Read the model definition and answer for the solid it produces. Units are mm, in the model's axes. Coordinates: 2 decimals unless noted, no trailing zeros. Write each loop counter-clockwise with the first axis right and the second up, starting at its lowest first coordinate (ties: lowest second). Pieces come first, ordered by that corner, then holes. Notation, with made-up numbers: (80, 44.25) -> (118, 44.25) arc R19 ccw to (118, 80.25) -> close; hole circle Ø1 at (12.25, -13). An arc over 180 degrees is marked (long way). One line per item, written item: value. Start each with the question number.
1. Find section B-B, the plane x = -12.7. Write down the section's boundary in (y, z).
2. Find section A-A, the plane y = 0. Write down the section's boundary in (x, z).
3. For a pull along Y with two mould halves and no side action, classify faces 1 (the flat face through (0, -25.4, -3)), 2 (the flat face through (0, 25.4, -3)), 3 (the cylindrical face through (-9.59, 2.85, -5.4)), 4 (the flat face through (0, 0, 0)) as pulls with the +Y half, pulls with the -Y half, needs draft (parallel to the pull), parting line crosses it, or undercut.
4. Consider line 1 along X through (y, z) = (0, -4.75); line 2 along Y through (x, z) = (-12.7, -5.7); line 3 along X through (y, z) = (4, -2). Determine where each line is inside the solid, lowest interval first.
5. Find section C-C, the plane z = -1.25. Write down the section's boundary in (x, y), and give its area (3 significant figures).
6. Given P1, Ø13.5, axis at x = -12.7, y = 0, coming from the -Z side; P2, Ø5, axis at x = 12.7, y = 0, coming from the +Z side, each flat-ended and moving along its own axis, determine where each tip first touches the part or whether it passes through.
```python
from build123d import *

# Parameters (mm, degrees)
SKETCH1_W                                         = 50.8
SKETCH1_H                                         = 50.8
SKETCH1_R                                         = 3.2639
BOSS_EXTRUDE1_DEPTH                               = 6.35
CSK_FOR_5_16_FLAT_HEAD_MACHINE_SCREW1_D           = 8.4328
CSK_FOR_5_16_FLAT_HEAD_MACHINE_SCREW1_DEPTH       = 32.766
CSK_FOR_5_16_FLAT_HEAD_MACHINE_SCREW1_CSINK_D     = 16.129
CSK_FOR_5_16_FLAT_HEAD_MACHINE_SCREW1_CSINK_ANGLE = 82
CSK_FOR_5_16_FLAT_HEAD_MACHINE_SCREW1_TIP         = 2.533468714


with BuildPart() as part:
    # Sketch1 → Boss-Extrude1 (new body)
    with BuildSketch(Plane.XY):
        Rectangle(SKETCH1_W, SKETCH1_H)
        with Locations((-12.7, 0)):
            Circle(SKETCH1_R, mode=Mode.SUBTRACT)
        with Locations((12.7, 0)):
            Circle(SKETCH1_R, mode=Mode.SUBTRACT)
    extrude(amount=-BOSS_EXTRUDE1_DEPTH)

    # CSK for 5/16 Flat Head Machine Screw1
    with Locations(Plane(origin=(-12.7, 0, 0), x_dir=(1, 0, 0), z_dir=(0, 0, 1))):
        with Locations((0, 0), (25.4, 0)):
            CounterSinkHole(CSK_FOR_5_16_FLAT_HEAD_MACHINE_SCREW1_D / 2, CSK_FOR_5_16_FLAT_HEAD_MACHINE_SCREW1_CSINK_D / 2, depth=CSK_FOR_5_16_FLAT_HEAD_MACHINE_SCREW1_DEPTH, counter_sink_angle=CSK_FOR_5_16_FLAT_HEAD_MACHINE_SCREW1_CSINK_ANGLE)
            with Locations((0, 0, -(CSK_FOR_5_16_FLAT_HEAD_MACHINE_SCREW1_DEPTH + CSK_FOR_5_16_FLAT_HEAD_MACHINE_SCREW1_TIP / 2))):  # 118° drill point
                Cone(0, CSK_FOR_5_16_FLAT_HEAD_MACHINE_SCREW1_D / 2, CSK_FOR_5_16_FLAT_HEAD_MACHINE_SCREW1_TIP, mode=Mode.SUBTRACT)


solid = part.part
```
Answer block:
1. outline: (-25.4, -6.35) -> (-4.22, -6.35) -> (-4.22, -4.43) -> (-8.06, 0) -> (-25.4, 0) -> close; (4.22, -6.35) -> (25.4, -6.35) -> (25.4, 0) -> (8.06, 0) -> (4.22, -4.43) -> close
2. outline: (-25.4, -6.35) -> (-16.92, -6.35) -> (-16.92, -4.43) -> (-20.76, 0) -> (-25.4, 0) -> close; (-8.48, -6.35) -> (8.48, -6.35) -> (8.48, -4.43) -> (4.64, 0) -> (-4.64, 0) -> (-8.48, -4.43) -> close; (16.92, -6.35) -> (25.4, -6.35) -> (25.4, 0) -> (20.76, 0) -> (16.92, -4.43) -> close
3. face 1: pulls with the -Y half
3. face 2: pulls with the +Y half
3. face 3: undercut
3. face 4: needs draft
4. line 1: x = -25.4 to -16.92, -8.48 to 8.48, 16.92 to 25.4
4. line 2: y = -25.4 to -4.22, 4.22 to 25.4
4. line 3: x = -25.4 to -17.6, -7.8 to 7.8, 17.6 to 25.4
5. outline: (-25.4, -25.4) -> (25.4, -25.4) -> (25.4, 25.4) -> (-25.4, 25.4) -> close; hole circle Ø13.96 at (-12.7, 0); hole circle Ø13.96 at (12.7, 0)
5. area: 2,270 mm2
6. P1: stops at z = -6.35
6. P2: passes through
